Autodesk Inventor part; units mm, degrees
ref_plane "YZ Plane" through (0, 0, 0) normal (1, 0, 0) x (0, 1, 0)
ref_plane "XZ Plane" through (0, 0, 0) normal (0, 1, 0) x (-1, 0, 0)
ref_plane "XY Plane" through (0, 0, 0) normal (0, 0, 1) x (1, 0, 0)
sketch "スケッチ1" plane through (0, 0, 0) normal (0, 0, 1) x (1, 0, 0)
  line L0 (0, 0) -> (-92, 0) construction
  line L1 (0, 5) -> (-92, 5)
  line L2 (-92, -5) -> (0, -5)
  arc A0 (0, -5) -> (0, 5) centre (0, 0) ccw
  circle A1 centre (0, 0) radius 1.6
  line L3 (-29.5, 1.5) -> (-29.5, 6.5)
  line L4 (-29.5, 1.5) -> (17.5, 13.0396)
  line L5 (17.5, 13.0396) -> (17.5, 18.1985)
  line L6 (17.5, 18.1985) -> (-29.5, 6.5)
  circle A2 centre (0, 15) radius 1.5
  line L7 (0, 15) -> (0, 0)
  circle A3 centre (0, 15) radius 2.5
  circle A4 centre (15, 15) radius 2.5
  circle A5 centre (15, 15) radius 1.5
  line L8 (-30, 6.8908) -> (-30, 0.8624)
  line L9 (-30, 0.8624) -> (18, 12.6475)
  line L10 (18, 12.6475) -> (18, 18.8382)
  line L11 (18, 18.8382) -> (-30, 6.8908)
  line L12 (-92, 5) -> (-92, -5)
  line L13 (0, 0) -> (-11, 0)
  line L14 (-11, 0) -> (-11, -3.5)
  line L15 (-11, 0) -> (-7.5, 0) construction
  line L16 (-11, -3.5) -> (0, -3.5)
  circle A6 centre (0, 0) radius 3.5
  line L17 (0, 5) -> (2.4995, 2.45)
  line L18 (-11, 0) -> (-11, -5)
  line L19 (15, 15) -> (15, 15)
  circle A7 centre (15, 15) radius 1.5
  circle A8 centre (15, 15) radius 2.5
  line L20 (-67.5, 5) -> (-67.5, -5)
  point P0 (-15.2447, 5)
  point P1 (-29.5, 5)
  point P2 (0, 12.5)
  point P3 (0.6029, 12.5738)
  point P4 (0, 8.7429)
  point P5 (2.4387, 14.4497)
  point P6 (-1.8962, 13.3707)
  point P7 (-13.1477, 5)
  point P8 (-30, 5)
  point P9 (-11, -4.9654)
  dimension "d14" = 10
  dimension "d1" = 92
  dimension "d2" = 3.2
  dimension "d3" = 5
  dimension "d4" = 3
  dimension "d5" = 15
  dimension "d6" = 1
  dimension "d11" = 15
  dimension "d16" = 0.5
  dimension "d24" = 5
  dimension "d25" = 11
  dimension "d26" = 90
  dimension "d27" = 7
  dimension "d30" = 0
  dimension "d31" = 3
  dimension "d32" = 1
  dimension "d33" = 62
  dimension "d34" = 37.5
  dimension "d46" = 92
  dimension "d47" = 3.5
extrude "押し出し1" add sketch "スケッチ1" along normal blind 5 contours L20 L2 L12 L1 | L1 L8 L9 L7 A6 L13 L14 L18 L2 L20 | L14 L13 A6 L16 | L17 A6 L7 | A6 L13 A1 L7 | L7 A1 L13 A6
fillet "フィレット1" radius 5 2 edges at (-92, 5, 2.5) (-92, -5, 2.5)
fillet "フィレット2" radius 5 1 edges at (-13.1477, 5, 2.5)
sketch "スケッチ3" plane through (0, 0, 5) normal (0, 0, 1) x (1, 0, 0)
  arc A0 (-12.5429, 5) -> (-13.7351, 4.8558) centre (-12.5429, 0) ccw
  line L0 (-13.7351, 4.8558) -> (-30, 0.8624)
  line L1 (-30, 0.8624) -> (-30, 5)
  line L2 (-30, 5) -> (-87, 5)
  arc A1 (-87, 5) -> (-87, -5) centre (-87, 0) ccw
  line L3 (-87, -5) -> (-11, -5)
  line L4 (-11, -5) -> (-11, -3.5)
  line L5 (-11, -3.5) -> (0, -3.5)
  arc A2 (0, -3.5) -> (2.4995, 2.45) centre (0, 0) ccw
  line L6 (2.4995, 2.45) -> (0, 5)
  line L7 (0, 5) -> (-12.5429, 5)
  circle A3 centre (0, 0) radius 1.6
  circle A4 centre (-76, 0) radius 1.25
  dimension "d49" = 2.5
  dimension "d50" = 11
extrude "押し出し3" cut sketch "スケッチ3" against normal blind 10 contours A4
thread "ねじ3"
properties part number "カウンター" material "ポリカーボネート、スモーク"
The model under review builds one solid part; all positions refer to its coordinate system, in mm. A direction names the side the tool comes from. Round coordinates to 2 decimals unless told otherwise and drop trailing zeros. Loops run counter-clockwise (first coordinate to the right, second up) from the corner with the lowest first, then second, coordinate; pieces in that order, holes last. Notation, with made-up numbers: (88, -17.75) -> (141, -17.75) arc R10 cw to (141, -8.75) -> close; hole circle Ø5 at (76.25, -36). An arc over 180 degrees is marked (long way). Write item = value, one per line. Start each with the question number.
Item 1: Mouldability with a two-part tool opening along X and no side actions: class faces 4 (the cylindrical face through (-1.27, 0.97, 2.46)), 5 (the flat face through (-45, 0, 0)), 6 (the flat face through (1.232, 3.743, 2.465)) as released by +X, released by -X, zero draft, split by the parting line, or undercut.
Item 2: Insertion check: pin 1 (2.5 mm diameter, centred on x = -7, z = 2.5, fed in from -Y); pin 2 (1 mm diameter, centred on y = -3, z = 3.5, fed in from +X); pin 3 (2 mm diameter, centred on y = 2.5, z = 3.5, fed in from +X). Each pin has a flat end and moves straight along its axis. Give the tip position at first contact, or say it passes through.
Item 3: Take a section at B-B on x = -76. Give the boundary of the cut face in (y, z).
Item 4: For faces 1 (the flat face through (-6, -3.5, 2)), 2 (the cylindrical face through (-91, -3, 3)), 3 (the flat face through (-30, 3, 2)), list the 3-axis set-ups (+Z, -Z, +X, -X, +Y, -Y) from which the entire face can be reached by the end or side of a thin tool; tool diameter is ignored.
Item 5: To check wall thickness, follow L1, parallel to Y at x = -76, z = 2.75; L2, parallel to Y at x = 0, z = 3.1; L3, parallel to Y at x = -5, z = 4.4. State the ranges of each line that lie inside material, in increasing order.
Item 6: Take a section at C-C on x = -19. Give the boundary of the cut face in (y, z), plus the area to 3 significant figures.
Item 7: Take a section at A-A on z = 2.9. Count the separate pieces of the cut face and the enclosed holes in it, plus the area to 3 significant figures.
Result:
q1.face_4 = undercut
q1.face_5 = zero draft
q1.face_6 = released by +X
q2.pin_1 = -3.5
q2.pin_2 = 2.45
q2.pin_3 = 3.16
q3.outline = (-5, 0) -> (-1.25, 0) -> (-1.25, 5) -> (-5, 5) -> close; (1.25, 0) -> (5, 0) -> (5, 5) -> (1.25, 5) -> close
q4.face_1 = +Z, -Z, +X, -Y
q4.face_2 = +Z, -Z, -X, -Y
q4.face_3 = +Z, -Z, +Y
q5.L1 = -5 to -1.25, 1.25 to 5
q5.L2 = -3.5 to -1.6, 1.6 to 5
q5.L3 = -3.5 to 5
q6.outline = (-5, 0) -> (3.56, 0) -> (3.56, 5) -> (-5, 5) -> close
q6.area = 42.8 mm²
q7.separate_pieces = 1
q7.enclosed_holes = 2
q7.area = 866 mm²
